The model under review builds one solid part; all positions refer to its coordinate system, in mm. A direction names the side the tool comes from. Coordinates: 2 decimals unless noted, no trailing zeros. Loops run counter-clockwise (first coordinate to the right, second up) from the corner with the lowest first, then second, coordinate; pieces in that order, holes last. Notation, with made-up numbers: (76.5, 9) -> (129.5, 9) arc R24 ccw to (129.5, 22) -> close; hole circle Ø9 at (21.25, -29.5). An arc over 180 degrees is marked (long way). One line per question, with ' | ' between items. Start each with the question number.
from build123d import *

# Parameters (mm, degrees)
RESSALTO_EXTRUS_O1_DEPTH                = 6
CORTE_EXTRUS_O1_DEPTH                   = 100
CORTE_EXTRUS_O2_DEPTH                   = 100
CORTE_EXTRUS_O3_DEPTH                   = 100
FILETE1_R                               = 0.1
CORTE_EXTRUS_O4_DEPTH                   = 100
BROCA_DE_ROSQUEAR_PARA_TARRAXA_DE_M31_D = 2.5
ESBO_O9_W                               = 15
ESBO_O9_H                               = 8
CORTE_EXTRUS_O5_DEPTH                   = 3
ESBO_O10_W                              = 5
ESBO_O10_H                              = 8
CORTE_EXTRUS_O6_DEPTH                   = 3
BROCA_DE_ROSQUEAR_PARA_TARRAXA_DE_M21_D = 1.6
BROCA_DE_ROSQUEAR_PARA_TARRAXA_DE_M32_D = 2.5
ESBO_O15_W                              = 56.265856886
ESBO_O15_H                              = 5.410018906
CORTE_EXTRUS_O7_DEPTH                   = 5
ESBO_O16_W                              = 22
ESBO_O16_H                              = 2
CORTE_EXTRUS_O8_DEPTH                   = 10
CORTE_EXTRUS_O9_DEPTH                   = 100


with BuildPart() as part:
    # Esboço1 → Ressalto-extrusão1 (new body)
    with BuildSketch(Plane.XY):
        Polygon((0, 62), (22, 62), (22, 96), (78, 96), (78, 62), (100, 62), (100, 0), (0, 0), align=None)
    extrude(amount=RESSALTO_EXTRUS_O1_DEPTH)

    # Esboço2 → Corte-extrusão1 (cut)
    with BuildSketch(Plane.ZY):
        Polygon((0, 0), (2.702851981, 12.71591881), (4.274929738, 12.381763367), (4.34595667, 12.71591881), (6, 12.71591881), (6, 0), align=None)
    extrude(amount=-CORTE_EXTRUS_O1_DEPTH, mode=Mode.SUBTRACT)

    # Esboço3 → Corte-extrusão2 (cut)
    with BuildSketch(Plane(origin=(78, 0, 0), x_dir=(0, 0, -1), z_dir=(1, 0, 0))):
        Polygon((-6, 91.5), (0, 85.5), (0, 96), (-6, 96), align=None)
    extrude(amount=-CORTE_EXTRUS_O2_DEPTH, mode=Mode.SUBTRACT)

    # Esboço4 → Corte-extrusão3 (cut)
    with BuildSketch(Plane(origin=(100, 0, 0), x_dir=(0, 0, -1), z_dir=(1, 0, 0))):
        Polygon((-3.876629102, 12.466424781), (-6, 11.831800832), (-6, 13.966424781), align=None)
    extrude(amount=-CORTE_EXTRUS_O3_DEPTH, mode=Mode.SUBTRACT)

    # Filete1
    filete1_edges = [part.edges().sort_by_distance(p)[0] for p in [
        (50, 0, 0),
    ]]
    fillet(filete1_edges, radius=FILETE1_R)

    # Esboço5 → Corte-extrusão4 (cut)
    with BuildSketch(Plane.XY.offset(6)):
        Polygon((0, 12.466424781), (1.313793103, 0.168697266), (0, 0.851436445), align=None)
        Polygon((100, 12.466424781), (98.686206897, 0.168697266), (100, 0.851436445), align=None)
    extrude(amount=-CORTE_EXTRUS_O4_DEPTH, mode=Mode.SUBTRACT)

    # Broca de rosquear para tarraxa de M31 (through all)
    with Locations(Plane.XY.offset(6)):
        with Locations((92, 56.966424781), (92, 28.520905026), (8, 56.966424781), (8, 28.520905026)):
            Hole(BROCA_DE_ROSQUEAR_PARA_TARRAXA_DE_M31_D / 2)

    # Esboço9 → Corte-extrusão5 (cut)
    with BuildSketch(Plane.XY.offset(6)):
        with Locations((10.5, 20.966424781)):
            Rectangle(ESBO_O9_W, ESBO_O9_H)
        with Locations((89.5, 20.966424781)):
            Rectangle(ESBO_O9_W, ESBO_O9_H)
    extrude(amount=-CORTE_EXTRUS_O5_DEPTH, mode=Mode.SUBTRACT)

    # Esboço10 → Corte-extrusão6 (cut)
    with BuildSketch(Plane(origin=(0, 0, 0), x_dir=(-1, 0, 0), z_dir=(0, 0, -1))):
        with Locations((-90, 20.966424781)):
            Rectangle(ESBO_O10_W, ESBO_O10_H)
        with Locations((-10, 20.966424781)):
            Rectangle(ESBO_O10_W, ESBO_O10_H)
    extrude(amount=-CORTE_EXTRUS_O6_DEPTH, mode=Mode.SUBTRACT)

    # Broca de rosquear para tarraxa de M21 (through all)
    with Locations(Plane.XY.offset(3)):
        with Locations((5.4999996, 20.966424401), (94.5000004, 20.966425161)):
            Hole(BROCA_DE_ROSQUEAR_PARA_TARRAXA_DE_M21_D / 2)

    # Broca de rosquear para tarraxa de M32 (through all)
    with Locations(Plane(origin=(0, 0, 0), x_dir=(-1, 0, 0), z_dir=(0, 0, -1))):
        with Locations((-30.75, 66), (-69.25, 66), (-69.25, 87.551471863), (-30.75, 87.551471863)):
            Hole(BROCA_DE_ROSQUEAR_PARA_TARRAXA_DE_M32_D / 2)

    # Esboço15 → Corte-extrusão7 (cut)
    with BuildSketch(Plane.XY.offset(6)):
        with Locations((50.132928443, 92.756481316)):
            Rectangle(ESBO_O15_W, ESBO_O15_H)
    extrude(amount=-CORTE_EXTRUS_O7_DEPTH, mode=Mode.SUBTRACT)

    # Esboço16 → Corte-extrusão8 (cut)
    with BuildSketch(Plane(origin=(0, 0, 0), x_dir=(-1, 0, 0), z_dir=(0, 0, -1))):
        with Locations((-11, 61)):
            Rectangle(ESBO_O16_W, ESBO_O16_H)
        with Locations((-89, 61)):
            Rectangle(ESBO_O16_W, ESBO_O16_H)
    extrude(amount=-CORTE_EXTRUS_O8_DEPTH, mode=Mode.SUBTRACT)

    # Esboço17 → Corte-extrusão9 (cut)
    with BuildSketch(Plane.ZY):
        Polygon((0.623735072, 2.934442802), (0, 3.067021785), (0, 0), align=None)
    extrude(amount=-CORTE_EXTRUS_O9_DEPTH, mode=Mode.SUBTRACT)


solid = part.part
1) Wall thickness on L1, parallel to X at y = 66, z = 2.55; L2, parallel to X at y = 68.5, z = 3.35; L3, parallel to Y at x = 91, z = 5.6: over which ranges is each line inside the solid? List them lowest first.
2) Machinability: for faces 1 (the face through (0.39, 8.83, 1.05)), 2 (the face through (12.5, 21, 1)), 3 (the face through (82, 21, 5)), which of the approach directions +Z, -Z, +X, -X, +Y, -Y give a long, thin tool a straight path to every point of the face, cutting with its end or side? Answer none if there is none.
3) Consider section A-A, the plane y = 66. Write out the cut boundary in (x, z), plus the area to 3 significant figures.
4) Insertion check: pin 1 Ø2 at (x, y) = (30.75, 87.55) entering from -Z; pin 2 Ø1.5 at (y, z) = (20.5, 5) entering from -X; pin 3 Ø3 at (y, z) = (76.5, 4) entering from -X; pin 4 Ø1.5 at (x, y) = (21.5, 12.5) entering from +Z. Each pin has a flat end and moves straight along its axis. Give the tip position at first contact, or say it passes through.
5) Mouldability with a two-part tool opening along X and no side actions: class faces 4 (the face through (99.61, 8.83, 1.05)), 5 (the face through (89, 60, 3)), 6 (the face through (90, 24.966, 4)) as +X half, -X half, draft (parallel to the pull), parting line (faces both ways), or undercut.
6) Consider section B-B, the plane x = 30.75. Write out the cut boundary in (y, z), plus the area to 3 significant figures.
Filled sheet:
1) L1: 22 to 29.5, 32 to 68, 70.5 to 78 | L2: 22 to 78 | L3: 13.68 to 16.97, 24.97 to 27.77, 29.27 to 56.22, 57.72 to 60
2) face 1: +Z, -Z, -X, -Y | face 2: +Z, -Z | face 3: +Z
3) outline: (22, 0) -> (29.5, 0) -> (29.5, 6) -> (22, 6) -> close; (32, 0) -> (68, 0) -> (68, 6) -> (32, 6) -> close; (70.5, 0) -> (78, 0) -> (78, 6) -> (70.5, 6) -> close | area: 306 mm^2
4) pin 1: through | pin 2: x = 0 | pin 3: x = 22 | pin 4: z = 4.99
5) face 4: +X half | face 5: draft | face 6: undercut
6) outline: (2.93, 0.62) -> (3.07, 0) -> (64.75, 0) -> (64.75, 6) -> (13.97, 6) -> (12.47, 3.88) -> (12.72, 2.7) -> close; (67.25, 0) -> (85.5, 0) -> (86.3, 0.8) -> (86.3, 6) -> (67.25, 6) -> close; (88.8, 3.3) -> (90.05, 4.55) -> (90.05, 6) -> (88.8, 6) -> close | area: 444 mm^2
